from build123d import *

# Parameters (mm, degrees)
EXTRUDE1_DEPTH                                   = 6.35
CBORE_FOR_1_4_SOCKET_HEAD_CAP_SCREW1_D           = 6.7564
CBORE_FOR_1_4_SOCKET_HEAD_CAP_SCREW1_DEPTH       = 9.525
CBORE_FOR_1_4_SOCKET_HEAD_CAP_SCREW1_CBORE_D     = 11.1125
CBORE_FOR_1_4_SOCKET_HEAD_CAP_SCREW1_CBORE_DEPTH = 6.35
F_1_4_20_TAPPED_HOLE1_D                          = 5.1054
CBORE_FOR_1_4_SOCKET_HEAD_CAP_SCREW3_D           = 6.7564
CBORE_FOR_1_4_SOCKET_HEAD_CAP_SCREW3_DEPTH       = 9.525
CBORE_FOR_1_4_SOCKET_HEAD_CAP_SCREW3_CBORE_D     = 11.1125
CBORE_FOR_1_4_SOCKET_HEAD_CAP_SCREW3_CBORE_DEPTH = 6.35
F_1_4_20_TAPPED_HOLE4_D                          = 5.1054
CBORE_FOR_1_4_SOCKET_HEAD_CAP_SCREW6_D           = 6.7564
CBORE_FOR_1_4_SOCKET_HEAD_CAP_SCREW6_DEPTH       = 9.525
CBORE_FOR_1_4_SOCKET_HEAD_CAP_SCREW6_CBORE_D     = 11.1125
CBORE_FOR_1_4_SOCKET_HEAD_CAP_SCREW6_CBORE_DEPTH = 6.35
F_1_4_20_TAPPED_HOLE7_D                          = 5.1054
FILLET1_R                                        = 3.175


with BuildPart() as part:
    # Sketch1 → Extrude1 (new, symmetric)
    with BuildSketch(Plane.XY):
        with BuildLine():
            Line((-39.6875, 88.9), (-39.6875, 0))
            ThreePointArc((-39.6875, 0), (-32.485618813, -22.798733003), (-13.49375, -37.323134477))
            Line((-13.49375, -37.323134477), (-13.49375, -56.373134477))
            Line((-13.49375, -56.373134477), (-3.96875, -56.373134477))
            Line((-3.96875, -56.373134477), (-3.96875, -36.296166184))
            ThreePointArc((-3.96875, -36.296166184), (0, 36.5125), (3.96875, -36.296166184))
            Line((3.96875, -36.296166184), (3.96875, -56.373134477))
            Line((3.96875, -56.373134477), (13.49375, -56.373134477))
            Line((13.49375, -56.373134477), (13.49375, -37.323134477))
            ThreePointArc((13.49375, -37.323134477), (14.978378625, -36.752494201), (16.438950589, -36.122826022))
            Line((16.438950589, -36.122826022), (101.793886149, 2.72091138))
            ThreePointArc((101.793886149, 2.72091138), (117.234328534, 14.176693941), (126.619887312, 30.95625))
            Line((126.619887312, 30.95625), (145.669887312, 30.95625))
            Line((145.669887312, 30.95625), (145.669887312, 40.48125))
            Line((145.669887312, 40.48125), (124.142537174, 40.48125))
            ThreePointArc((124.142537174, 40.48125), (41.274610429, 44.45), (124.142537174, 48.41875))
            Line((124.142537174, 48.41875), (145.669887312, 48.41875))
            Line((145.669887312, 48.41875), (145.669887312, 57.94375))
            Line((145.669887312, 57.94375), (126.619887312, 57.94375))
            ThreePointArc((126.619887312, 57.94375), (117.234328534, 74.723306059), (101.793886149, 86.17908862))
            Line((101.793886149, 86.17908862), (16.438950589, 125.022826022))
            ThreePointArc((16.438950589, 125.022826022), (14.978378625, 125.652494201), (13.49375, 126.223134477))
            Line((13.49375, 126.223134477), (13.49375, 145.273134477))
            Line((13.49375, 145.273134477), (3.96875, 145.273134477))
            Line((3.96875, 145.273134477), (3.96875, 125.196166184))
            ThreePointArc((3.96875, 125.196166184), (0, 52.3875), (-3.96875, 125.196166184))
            Line((-3.96875, 125.196166184), (-3.96875, 145.273134477))
            Line((-3.96875, 145.273134477), (-13.49375, 145.273134477))
            Line((-13.49375, 145.273134477), (-13.49375, 126.223134477))
            ThreePointArc((-13.49375, 126.223134477), (-32.485618813, 111.698733003), (-39.6875, 88.9))
        make_face()
    extrude(amount=EXTRUDE1_DEPTH, both=True)

    # CBORE for 1/4 Socket Head Cap Screw1
    with Locations(Plane(origin=(13.49375, 0, 0), x_dir=(0, 0, -1), z_dir=(1, 0, 0))):
        with Locations((0, 135.748134477)):
            CounterBoreHole(CBORE_FOR_1_4_SOCKET_HEAD_CAP_SCREW1_D / 2, CBORE_FOR_1_4_SOCKET_HEAD_CAP_SCREW1_CBORE_D / 2, CBORE_FOR_1_4_SOCKET_HEAD_CAP_SCREW1_CBORE_DEPTH, depth=CBORE_FOR_1_4_SOCKET_HEAD_CAP_SCREW1_DEPTH)

    # 1/4-20 Tapped Hole1 (through all)
    with Locations(Plane(origin=(-3.96875, 0, 0), x_dir=(0, 0, -1), z_dir=(1, 0, 0))):
        with Locations((0, 135.748134477)):
            Hole(F_1_4_20_TAPPED_HOLE1_D / 2)

    # CBORE for 1/4 Socket Head Cap Screw3
    with Locations(Plane(origin=(13.49375, 0, 0), x_dir=(0, 0, -1), z_dir=(1, 0, 0))):
        with Locations((0, -46.848134477)):
            CounterBoreHole(CBORE_FOR_1_4_SOCKET_HEAD_CAP_SCREW3_D / 2, CBORE_FOR_1_4_SOCKET_HEAD_CAP_SCREW3_CBORE_D / 2, CBORE_FOR_1_4_SOCKET_HEAD_CAP_SCREW3_CBORE_DEPTH, depth=CBORE_FOR_1_4_SOCKET_HEAD_CAP_SCREW3_DEPTH)

    # 1/4-20 Tapped Hole4 (through all)
    with Locations(Plane(origin=(-3.96875, 0, 0), x_dir=(0, 0, -1), z_dir=(1, 0, 0))):
        with Locations((0, -46.848134477)):
            Hole(F_1_4_20_TAPPED_HOLE4_D / 2)

    # CBORE for 1/4 Socket Head Cap Screw6
    with Locations(Plane(origin=(0, 57.94375, 0), x_dir=(1, 0, 0), z_dir=(0, 1, 0))):
        with Locations((136.144887312, 0)):
            CounterBoreHole(CBORE_FOR_1_4_SOCKET_HEAD_CAP_SCREW6_D / 2, CBORE_FOR_1_4_SOCKET_HEAD_CAP_SCREW6_CBORE_D / 2, CBORE_FOR_1_4_SOCKET_HEAD_CAP_SCREW6_CBORE_DEPTH, depth=CBORE_FOR_1_4_SOCKET_HEAD_CAP_SCREW6_DEPTH)

    # 1/4-20 Tapped Hole7 (through all)
    with Locations(Plane(origin=(0, 40.48125, 0), x_dir=(1, 0, 0), z_dir=(0, 1, 0))):
        with Locations((136.144887312, 0)):
            Hole(F_1_4_20_TAPPED_HOLE7_D / 2)

    # Fillet1
    fillet1_edges = [part.edges().sort_by_distance(p)[0] for p in [
        (-13.49375, 126.223134477, 0),
        (13.49375, 126.223134477, 0),
        (126.619887312, 57.94375, 0),
        (126.619887312, 30.95625, 0),
        (13.49375, -37.323134477, 0),
        (-13.49375, -37.323134477, 0),
    ]]
    fillet(fillet1_edges, radius=FILLET1_R)


solid = part.part
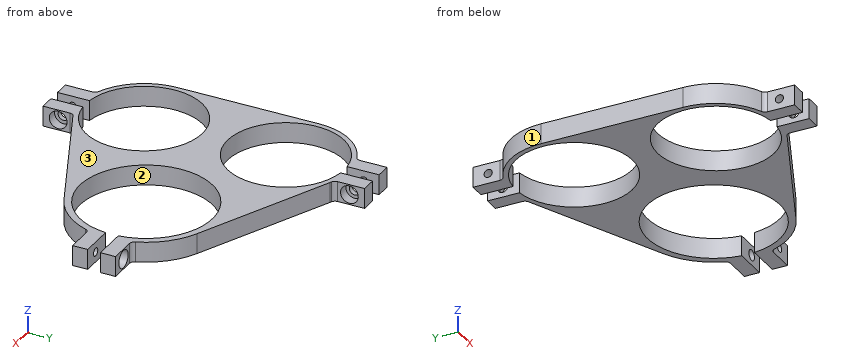
Input: part model. Units: mm. Frame: model coordinates. Face numbers are marked on the shaded views. Round coordinates to 2 decimals unless told otherwise and drop trailing zeros. Write each loop counter-clockwise with the first axis right and the second up, starting at its lowest first coordinate (ties: lowest second). Pieces come first, ordered by that corner, then holes.
1) Cut plane D-D (z = 0). Count the separate pieces of the cut face and the enclosed holes in it, then the cut area to 3 significant figures.
2) Cut plane B-B (x = 115.5). Return the cut outline in (y, z).
3) Contact query for flat-ended pins moving along their axis: P1, Ø1, axis at x = 33, z = 0, coming from the +Y side; P2, Ø1.5, axis at x = 122, z = -3.5, coming from the +Y side; P3, Ø3, axis at x = 88.5, z = -2.5, coming from the +Y side. Output: stop coordinate, or through.
4) Cut plane C-C (y = 118). Return the cut outline in (x, z), then the cut area to 3 significant figures.
5) Ray query, L1, parallel to X at y = 129.5, z = 5.25; L2, parallel to X at y = 75, z = -4.5; L3, parallel to Y at x = -6.5, z = 0. Return the intervals inside material, ascending.
6) Draft query along Y for the marked faces 1, 2 and 3. Return one class per face: pulls with the +Y half, pulls with the -Y half, needs draft (parallel to the pull), parting line crosses it, or undercut.
7) Cut plane A-A (y = 68). Return the cut outline in (x, z).
Geometry says:
1. separate pieces: 7
1. enclosed holes: 0
1. area: 7,500 mm2
2. outline: (12.31, -6.35) - (18.85, -6.35) - (18.85, 6.35) - (12.31, 6.35) - close; (70.05, -6.35) - (76.59, -6.35) - (76.59, 6.35) - (70.05, 6.35) - close
3. P1: stops at y = 117.71
3. P2: stops at y = 69.43
3. P3: stops at y = 92.91
4. outline: (-26.99, -6.35) - (-22.05, -6.35) - (-22.05, 6.35) - (-26.99, 6.35) - close; (22.05, -6.35) - (31.87, -6.35) - (31.87, 6.35) - (22.05, 6.35) - close
4. area: 187 mm2
5. L1: x = -13.49 to -3.97, 3.97 to 13.49
5. L2: x = -39.69 to -33.76, 33.76 to 54.67, 110.93 to 116.99
5. L3: y = -56.37 to -49.4, -44.3 to -35.93, 35.93 to 52.97, 124.83 to 133.2, 138.3 to 145.27
6. face 1: pulls with the +Y half
6. face 2: undercut
6. face 3: needs draft
7. outline: (-39.69, -6.35) - (-29.94, -6.35) - (-29.94, 6.35) - (-39.69, 6.35) - close; (29.94, -6.35) - (48.6, -6.35) - (48.6, 6.35) - (29.94, 6.35) - close; (117.01, -6.35) - (122.14, -6.35) - (122.14, 6.35) - (117.01, 6.35) - close
